Here's how the part is built. I have some questions about the finished solid (model axes, mm). Face numbers are marked on the shaded views. A direction names the side the tool comes from. Give positions to 0.01 mm unless a question says otherwise; leave off trailing zeros. Write each loop counter-clockwise with the first axis right and the second up, starting at its lowest first coordinate (ties: lowest second). Pieces come first, ordered by that corner, then holes. Notation, with made-up numbers: (15, 35.25) -> (62, 35.25) arc R22 cw to (62, 70.25) -> close; hole circle Ø2 at (0.5, 36.25). An arc over 180 degrees is marked (long way). Answer as CSV lines item,"result". Start each with the question number.
from build123d import *
from build123d.topology import SkipClean

# Parameters (mm, degrees)
SKETCH1_R           = 11.5062
BOSS_EXTRUDE1_DEPTH = 4.7625
CUT_EXTRUDE1_START  = 4.7625
CUT_EXTRUDE1_DEPTH  = 1.5875
CUT_EXTRUDE2_START  = -3.175
CUT_EXTRUDE2_DEPTH  = 1.5875
FILLET1_R           = 1.5875


with BuildPart() as part:
    # Sketch1 → Boss-Extrude1 (new, symmetric)
    # profile 1 of 2: a face of its own
    with BuildSketch(Plane.XY):
        with BuildLine():
            ThreePointArc((-12.585193267, -7.559797873), (-10.89585042, -11.492870345), (-10.31875, -15.734319794))
            Line((-10.31875, -15.734319794), (-10.31875, -49.389319794))
            Line((-10.31875, -49.389319794), (10.31875, -49.389319794))
            Line((10.31875, -49.389319794), (10.31875, -37.783763396))
            Line((10.31875, -37.783763396), (16.282292064, -47.887675791))
            Line((16.282292064, -47.887675791), (34.055016522, -37.397839205))
            Line((34.055016522, -37.397839205), (16.883960941, -8.3052564))
            ThreePointArc((16.883960941, -8.3052564), (15.225065006, -4.359245427), (14.68076155, -0.11346257))
            ThreePointArc((14.68076155, -0.11346257), (3.867793812, -14.162549363), (-12.585193267, -7.559797873))
        make_face()
        with BuildLine():
            ThreePointArc((5.55625, -39.070569794), (0, -44.626819794), (-5.55625, -39.070569794))
            Line((-5.55625, -39.070569794), (-5.55625, -27.958069794))
            ThreePointArc((-5.55625, -27.958069794), (0, -22.401819794), (5.55625, -27.958069794))
            Line((5.55625, -27.958069794), (5.55625, -39.070569794))
        make_face(mode=Mode.SUBTRACT)
        with BuildLine():
            ThreePointArc((24.708700277, -30.932208496), (22.747922773, -38.541359546), (15.138771723, -36.580582042))
            Line((15.138771723, -36.580582042), (9.490398177, -27.010653488))
            ThreePointArc((9.490398177, -27.010653488), (11.451175681, -19.401502438), (19.060326731, -21.362279942))
            Line((19.060326731, -21.362279942), (24.708700277, -30.932208496))
        make_face(mode=Mode.SUBTRACT)
    # profile 2 of 2: a face of its own
    with BuildSketch(Plane.XY):
        with BuildLine():
            ThreePointArc((14.68076155, -0.11346257), (-3.867793812, 14.162549363), (-12.585193267, -7.559797873))
            ThreePointArc((-12.585193267, -7.559797873), (3.867793812, -14.162549363), (14.68076155, -0.11346257))
        make_face()
        with Locations(Location((0, 0, 0), (0, 0, 180))):
            Circle(SKETCH1_R, mode=Mode.SUBTRACT)
    extrude(amount=BOSS_EXTRUDE1_DEPTH, both=True)

    # Sketch3 → Cut-Extrude1 (cut)
    with SkipClean():  # the faces are left unmerged after this step: merging them gives an invalid solid
        with BuildSketch(Plane.XY.offset(CUT_EXTRUDE1_START)):
            with BuildLine():
                ThreePointArc((-12.585193267, -7.559797873), (3.867793812, -14.162549363), (14.68076155, -0.11346257))
                ThreePointArc((14.68076155, -0.11346257), (15.225065006, -4.359245427), (16.883960941, -8.3052564))
                Line((16.883960941, -8.3052564), (34.055016522, -37.397839205))
                Line((34.055016522, -37.397839205), (16.282292064, -47.887675791))
                Line((16.282292064, -47.887675791), (10.31875, -37.783763396))
                Line((10.31875, -37.783763396), (10.31875, -49.389319794))
                Line((10.31875, -49.389319794), (-10.31875, -49.389319794))
                Line((-10.31875, -49.389319794), (-10.31875, -15.734319794))
                ThreePointArc((-10.31875, -15.734319794), (-10.89585042, -11.492870345), (-12.585193267, -7.559797873))
            make_face()
            with BuildLine():
                ThreePointArc((19.060326731, -21.362279942), (11.451175681, -19.401502438), (9.490398177, -27.010653488))
                Line((9.490398177, -27.010653488), (15.138771723, -36.580582042))
                ThreePointArc((15.138771723, -36.580582042), (22.747922773, -38.541359546), (24.708700277, -30.932208496))
                Line((24.708700277, -30.932208496), (19.060326731, -21.362279942))
            make_face(mode=Mode.SUBTRACT)
            with BuildLine():
                ThreePointArc((5.55625, -27.958069794), (0, -22.401819794), (-5.55625, -27.958069794))
                Line((-5.55625, -27.958069794), (-5.55625, -39.070569794))
                ThreePointArc((-5.55625, -39.070569794), (0, -44.626819794), (5.55625, -39.070569794))
                Line((5.55625, -39.070569794), (5.55625, -27.958069794))
            make_face(mode=Mode.SUBTRACT)
        extrude(amount=-CUT_EXTRUDE1_DEPTH, mode=Mode.SUBTRACT)

    # Sketch3<11> → Cut-Extrude2 (cut)
    with SkipClean():  # the faces are left unmerged after this step: merging them gives an invalid solid
        with BuildSketch(Plane.XY.offset(CUT_EXTRUDE2_START)):
            with BuildLine():
                ThreePointArc((-12.585193267, -7.559797873), (3.867793812, -14.162549363), (14.68076155, -0.11346257))
                ThreePointArc((14.68076155, -0.11346257), (15.225065006, -4.359245427), (16.883960941, -8.3052564))
                Line((16.883960941, -8.3052564), (34.055016522, -37.397839205))
                Line((34.055016522, -37.397839205), (16.282292064, -47.887675791))
                Line((16.282292064, -47.887675791), (10.31875, -37.783763396))
                Line((10.31875, -37.783763396), (10.31875, -49.389319794))
                Line((10.31875, -49.389319794), (-10.31875, -49.389319794))
                Line((-10.31875, -49.389319794), (-10.31875, -15.734319794))
                ThreePointArc((-10.31875, -15.734319794), (-10.89585042, -11.492870345), (-12.585193267, -7.559797873))
            make_face()
            with BuildLine():
                ThreePointArc((19.060326731, -21.362279942), (11.451175681, -19.401502438), (9.490398177, -27.010653488))
                Line((9.490398177, -27.010653488), (15.138771723, -36.580582042))
                ThreePointArc((15.138771723, -36.580582042), (22.747922773, -38.541359546), (24.708700277, -30.932208496))
                Line((24.708700277, -30.932208496), (19.060326731, -21.362279942))
            make_face(mode=Mode.SUBTRACT)
            with BuildLine():
                ThreePointArc((5.55625, -27.958069794), (0, -22.401819794), (-5.55625, -27.958069794))
                Line((-5.55625, -27.958069794), (-5.55625, -39.070569794))
                ThreePointArc((-5.55625, -39.070569794), (0, -44.626819794), (5.55625, -39.070569794))
                Line((5.55625, -39.070569794), (5.55625, -27.958069794))
            make_face(mode=Mode.SUBTRACT)
        extrude(amount=-CUT_EXTRUDE2_DEPTH, mode=Mode.SUBTRACT)

    # Fillet1
    fillet1_edges = [part.edges().sort_by_distance(p)[0] for p in [
        (34.055016522, -37.397839205, 0),
        (16.282292064, -47.887675791, 0),
        (10.31875, -37.783763396, 0),
        (10.31875, -49.389319794, 0),
        (-10.31875, -49.389319794, 0),
    ]]
    fillet(fillet1_edges, radius=FILLET1_R)


solid = part.part
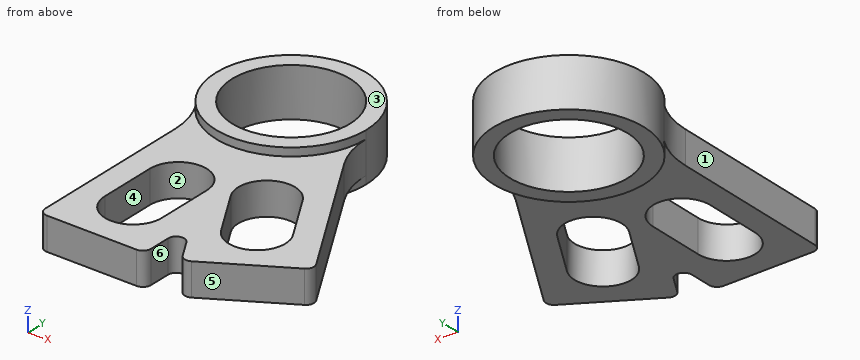
Item 1: If we section it at D-D (x = 27): Please give me the cut outline in (y, z) (3 decimals), and give its area (3 significant figures).
Item 2: I'm going to push flat-ended pins straight in: pin 1 (1.9 mm diameter, centred on y = -34.5, z = -0.5, fed in from -X); pin 2 (5 mm diameter, centred on x = 17.5, y = 7, fed in from +Z); pin 3 (14 mm diameter, centred on x = 9.5, y = -29, fed in from +Z) (3 decimals); pin 4 (10 mm diameter, centred on x = -3, y = -26.5, fed in from -Z) (3 decimals). Where does each tip first touch, or does it pass through?
Item 3: For the marked faces 1, 2 and 3, which set-ups out of +Z, -Z, +X, -X, +Y, -Y let a thin tool reach every point of the face, with its end or its side?
Item 4: We'd pull the mould along Y, two halves only. Please class the marked faces 4, 5 and 6: released by +Y, released by -Y, zero draft, split by the parting line, or undercut.
Item 5: If we section it at B-B (z = -1.25): State how many separate pieces and enclosed holes the cut face has, and give its area (3 significant figures).
Item 6: If we section it at C-C (y = -40.5): Please give me the cut outline in (x, z) (3 decimals).
Item 7: If I drill on line 1 (Y direction, x = 0, z = -2.5); line 2 (Y direction, x = 1.5, z = 2.25); line 3 (Y direction, x = -2.5, z = 4), over which ranges is the centre line in solid material (lowest first)? Write a range as [from, to].
Item 8: If we section it at A-A (x = 0): Please give me the cut outline in (y, z) (1 decimal), and give its area (3 significant figures).
Final values:
1,outline,"(-41.562, -3.175) -> (-25.445, -3.175) -> (-25.445, 3.175) -> (-41.562, 3.175) -> close"
1,area,"102 mm2"
2,pin 1,"x = -10.32"
2,pin 2,"through"
2,pin 3,"z = 3.175"
2,pin 4,"z = -3.175"
3,face 1,"+Z, -Z, -X, -Y"
3,face 2,"+Z, -Z"
3,face 3,"+Z, +X, -X, +Y, -Y"
4,face 4,"undercut"
4,face 5,"released by -Y"
4,face 6,"zero draft"
5,separate pieces,"1"
5,enclosed holes,"3"
5,area,"1,150 mm2"
6,outline,"(-10.319, -3.175) -> (-5.369, -3.175) -> (-5.369, 3.175) -> (-10.319, 3.175) -> close; (5.369, -3.175) -> (28.799, -3.175) -> (28.799, 3.175) -> (5.369, 3.175) -> close"
7,line 1,"[-49.39, -44.63], [-22.4, -11.51], [11.51, 14.68]"
7,line 2,"[-49.39, -44.42], [-22.61, -11.41], [11.41, 14.6]"
7,line 3,"[-14.47, -11.23], [11.23, 14.47]"
8,outline,"(-49.4, -3.2) -> (-44.6, -3.2) -> (-44.6, 3.2) -> (-49.4, 3.2) -> close; (-22.4, -3.2) -> (-14.7, -3.2) -> (-14.7, -4.8) -> (-11.5, -4.8) -> (-11.5, 4.8) -> (-14.7, 4.8) -> (-14.7, 3.2) -> (-22.4, 3.2) -> close; (11.5, -4.8) -> (14.7, -4.8) -> (14.7, 4.8) -> (11.5, 4.8) -> close"
8,area,"140 mm2"
